Here's how the part is built. I have some questions about the finished solid (model axes, mm). Give positions to 0.01 mm unless a question says otherwise; leave off trailing zeros. Order: outer loops, then holes, each group sorted by start corner. A loop starts at its lowest first (then second) coordinate and runs counter-clockwise, first axis right, second up.
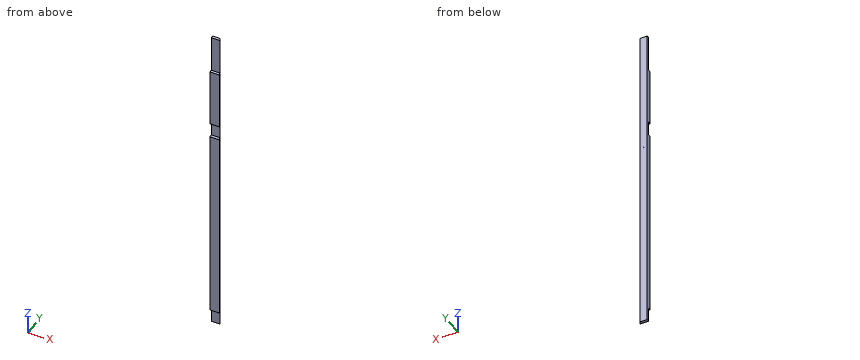
from build123d import *

# Parameters (mm, degrees)
F1_DEPTH = 1111.25
F2_W     = 122.435573
F2_H     = 50.8
F2_W_2   = 93.867282
F2_W_3   = 343.160421
F2_H_2   = 127
F3_DEPTH = 25.4
F4_R     = 0.79375
F5_DEPTH = 25.4


with BuildPart() as f1:
    # F0 (on Top) → F1 (new body)
    with BuildSketch(Plane.XY):
        Polygon((7.890768, -9.525), (0, 9.525), (-25.4, 9.525), (-25.4, -9.525), align=None)
    extrude(amount=F1_DEPTH)

    # F2 (on Front) → F3 (cut)
    with BuildSketch(Plane.XZ):
        with Locations((22.446524, 25.4)):
            Rectangle(F2_W, F2_H)
        with Locations((2.720783, 755.65)):
            Rectangle(F2_W_2, F2_H)
        with Locations((-38.781822, 1047.75)):
            Rectangle(F2_W_3, F2_H_2)
    extrude(amount=F3_DEPTH, mode=Mode.SUBTRACT)

    # F4 (on Front) → F5 (cut)
    with BuildSketch(Plane.XZ):
        with Locations((12.7, 101.6)):
            Circle(F4_R)
        with Locations((12.7, 155.575)):
            Circle(F4_R)
        with Locations((12.7, 625.475)):
            Circle(F4_R)
        with Locations((12.7, 679.45)):
            Circle(F4_R)
        with Locations((-12.7, 625.475)):
            Circle(F4_R)
        with Locations((-12.7, 679.45)):
            Circle(F4_R)
        with Locations((-12.7, 101.6)):
            Circle(F4_R)
        with Locations((-12.7, 155.575)):
            Circle(F4_R)
    extrude(amount=-F5_DEPTH, mode=Mode.SUBTRACT)


solid = f1.part
Q1. If we section it at B-B on z = 305: List the corners of the cut face in (x, y) for me (3 decimals).
Filled sheet:
outline: (-25.4, -9.525) - (7.891, -9.525) - (0, 9.525) - (-25.4, 9.525) - close
Q2. I'm going to push flat-ended pins straight in: P1, Ø10, axis at x = -18, y = -6.5, coming from the -Z side; P2, Ø1.3, axis at x = -12.7, z = 679.45, coming from the +Y side; P3, Ø9, axis at x = -15, z = 761, coming from the -Y side. Where does each tip first touch, or does it pass through?
Filled sheet:
P1: stops at z = 50.8
P2: stops at y = 0
P3: stops at y = 0
Q3. If we section it at A-A on y = 3.5: Give the number of separate pieces and of enclosed holes in the cut face, plus the area to 3 significant figures.
Filled sheet:
separate pieces: 1
enclosed holes: 4
area: 31,000 mm2
Q4. I need wall thicknesses on L1, parallel to Z at x = -12.7, y = 7; L2, parallel to X at y = 3.5, z = 101.6; L3, parallel to X at y = -1.75, z = 167. Which ranges of each line are inside material? Lowest first, please.
Filled sheet:
L1: z = 0 to 100.81, 102.39 to 154.78, 156.37 to 624.68, 626.27 to 678.66, 680.24 to 1111.25
L2: x = -25.4 to -13.49, -11.91 to 2.5
L3: x = -25.4 to 4.67
